Check sheet for the modelled part. Datum: model origin and axes. Units: mm. A direction names the side the tool comes from. Round coordinates to 2 decimals unless told otherwise and drop trailing zeros. Write each loop counter-clockwise with the first axis right and the second up, starting at its lowest first coordinate (ties: lowest second). Pieces come first, ordered by that corner, then holes.
Item 1: Section check A-A, the plane y = 0. Record the cut outline in (x, z).
Item 2: Set-up check for faces 4 (the flat face through (0, -23, 4)), 5 (the flat face through (4, 20, 4)), 6 (the flat face through (25.92, -14.11, -2.01)), 7 (the cylindrical face through (-25.148, 13.036, -1.93)): record each of +Z, -Z, +X, -X, +Y, -Y from which the full face is reachable in a straight line by a thin tool's end or side.
Item 3: Depth check by flat-ended pin: pin 1 (1.4 mm diameter, centred on y = -23, z = 2, fed in from -X); pin 2 (3.5 mm diameter, centred on x = -5.5, y = 21.5, fed in from -Z); pin 3 (5 mm diameter, centred on x = -3.5, y = -9.5, fed in from -Z); pin 4 (1.4 mm diameter, centred on x = 27.71, z = 1.7, fed in from -Y) (3 decimals). Enter the tip coordinate at first touch or a pass-through.
Item 4: Section check C-C, the plane z = -1.7. State how many separate pieces and enclosed holes the cut face has, plus the area to 3 significant figures.
Item 5: Release check for a two-part mould opening along Z. For faces 1 (the flat face through (5, 20, 6)), 2 (the cylindrical face through (-24.86, -13.036, 2.106)), 3 (the cylindrical face through (7.1, -17.6, 5)) record: pulls with the +Z half, pulls with the -Z half, needs draft (parallel to the pull), parting line crosses it, or undercut.
Item 6: Material ranges on line 1 along X through (y, z) = (13.5, -2); line 2 along X through (y, z) = (6, 0.25); line 3 along Y through (x, z) = (7.27, 5.6) (3 decimals), recorded low to high.
Item 7: Section check B-B, the plane x = -6.5. Record the cut outline in (y, z), plus the area to 3 significant figures.
from build123d import *

# Parameters (mm, degrees)
PAD_DEPTH       = 6.5
POCKET_DEPTH    = 6
SKETCH002_R     = 13.5
POCKET001_DEPTH = 1
SKETCH003_W     = 5.4
SKETCH003_H     = 6.5
PAD001_DEPTH    = 4.5
POCKET002_DEPTH = 10
SKETCH008_R     = 0.6
POCKET003_DEPTH = 2
SKETCH009_R     = 0.6
POCKET004_DEPTH = 2
FILLET_R        = 2.9
FILLET001_R     = 2.9
FILLET002_R     = 5
FILLET003_R     = 5
FILLET004_R     = 5
FILLET005_R     = 5
SKETCH010_W     = 3.95
SKETCH010_H     = 6.5
PAD002_DEPTH    = 4.5
POCKET005_DEPTH = 10
SKETCH012_R     = 0.6
POCKET006_DEPTH = 2
SKETCH013_R     = 0.6
POCKET007_DEPTH = 2
FILLET006_R     = 3.4
FILLET007_R     = 3.4
SKETCH014_R     = 20.45
SKETCH014_R_2   = 19.5
POCKET008_DEPTH = 0.3
SKETCH015_R     = 2.2
SKETCH015_R_2   = 0.975
PAD003_DEPTH    = 2
POCKET009_DEPTH = 4
POCKET010_DEPTH = 4
PAD004_DEPTH    = 3
CHAMFER_SIZE    = 2
CHAMFER001_SIZE = 2
CHAMFER002_SIZE = 2
CHAMFER003_SIZE = 2
SKETCH019_R     = 0.6
POCKET011_DEPTH = 2
SKETCH020_R     = 0.6
POCKET012_DEPTH = 2


with BuildPart() as part:
    # Sketch → Pad (new body)
    with BuildSketch(Plane.XY):
        with BuildLine():
            Line((-22.5019915649, 16), (-22.5019915649, -16))
            Line((-22.5019915649, -16), (-16.2858834577, -17.9000000001))
            ThreePointArc((-16.2858834577, -17.9000000001), (0.2206895737, -24.1989937004), (16.6096357576, -17.5999999999))
            Line((16.6096357576, -17.5999999999), (24.9082802252, -17.45))
            Line((24.9082802252, 17.45), (24.9082802252, -17.45))
            Line((16.6096357576, 17.6), (24.9082802252, 17.45))
            ThreePointArc((16.6096357576, 17.6), (0.2206895736, 24.1989937004), (-16.2858834578, 17.9))
            Line((-22.5019915649, 16), (-16.2858834578, 17.9))
        make_face()
    extrude(amount=PAD_DEPTH)

    # Sketch001 → Pocket (cut)
    with BuildSketch(Plane.XY):
        with BuildLine():
            Line((-14.8539557021, 16.9), (-21.2122180433, 15.55))
            Line((-21.2122180433, 15.55), (-21.2122180433, -15.55))
            Line((-21.2122180433, -15.55), (-14.8539557021, -16.9))
            ThreePointArc((-14.8539557021, -16.9), (-0.0760301383, -22.4998715423), (14.739402973, -17))
            Line((14.739402973, -17), (23.6191552218, -16.4))
            Line((23.6191552218, 16.4), (23.6191552218, -16.4))
            Line((14.739402973, 17), (23.6191552218, 16.4))
            ThreePointArc((14.739402973, 17), (-0.0760301383, 22.4998715423), (-14.8539557021, 16.9))
        make_face()
    extrude(amount=POCKET_DEPTH, mode=Mode.SUBTRACT)

    # Sketch002 (on Face19 of Pocket) → Pocket001 (cut)
    with BuildSketch(Plane(origin=(0, 0, 6), x_dir=(1, 0, 0), z_dir=(0, 0, -1))):
        Circle(SKETCH002_R)
    extrude(amount=-POCKET001_DEPTH, mode=Mode.SUBTRACT)

    # Sketch003 (on Face7 of Pad) → Pad001 (join)
    with BuildSketch(Plane.YZ.offset(24.9082802252)):
        with Locations((-14.75, 3.25)):
            Rectangle(SKETCH003_W, SKETCH003_H)
        with Locations((14.75, 3.25)):
            Rectangle(SKETCH003_W, SKETCH003_H)
    extrude(amount=PAD001_DEPTH)

    # Sketch006 (on Face22 of Pad001) → Pocket002 (cut)
    with BuildSketch(Plane.XY.offset(6.5)):
        with BuildLine():
            ThreePointArc((24.9082802252, 17.45), (26.9423471239, 15.7065020586), (29.4082802252, 14.6594169811))
            Line((29.4082802252, 17.45), (29.4082802252, 14.6594169811))
            Line((29.4082802252, 17.45), (24.9082802252, 17.45))
        make_face()
        with BuildLine():
            ThreePointArc((29.4082802252, -14.6594169811), (26.9423471239, -15.7065020586), (24.9082802252, -17.45))
            Line((29.4082802252, -17.45), (24.9082802252, -17.45))
            Line((29.4082802252, -14.6594169811), (29.4082802252, -17.45))
        make_face()
    extrude(amount=-POCKET002_DEPTH, mode=Mode.SUBTRACT)

    # Sketch008 (on Face27 of Pocket002) → Pocket003 (cut)
    with BuildSketch(Plane(origin=(0, -12.05, 0), x_dir=(-1, 0, 0), z_dir=(0, 1, 0))):
        with Locations((-27.7082802252, 1.7)):
            Circle(SKETCH008_R)
    extrude(amount=-POCKET003_DEPTH, mode=Mode.SUBTRACT)

    # Sketch009 (on Face26 of Pocket003) → Pocket004 (cut)
    with BuildSketch(Plane.XZ.offset(-12.05)):
        with Locations((27.7082802252, 1.7)):
            Circle(SKETCH009_R)
    extrude(amount=-POCKET004_DEPTH, mode=Mode.SUBTRACT)

    # Fillet
    fillet_edges = [part.edges().sort_by_distance(p)[0] for p in [
        (29.40828, -13.354708, 6.5),
    ]]
    fillet(fillet_edges, radius=FILLET_R)

    # Fillet001
    fillet001_edges = [part.edges().sort_by_distance(p)[0] for p in [
        (29.40828, 13.354708, 6.5),
    ]]
    fillet(fillet001_edges, radius=FILLET001_R)

    # Fillet002
    fillet002_edges = [part.edges().sort_by_distance(p)[0] for p in [
        (16.609636, -17.6, 3.25),
    ]]
    fillet(fillet002_edges, radius=FILLET002_R)

    # Fillet003
    fillet003_edges = [part.edges().sort_by_distance(p)[0] for p in [
        (16.609636, 17.6, 3.25),
    ]]
    fillet(fillet003_edges, radius=FILLET003_R)

    # Fillet004
    fillet004_edges = [part.edges().sort_by_distance(p)[0] for p in [
        (-16.285883, -17.9, 3.25),
    ]]
    fillet(fillet004_edges, radius=FILLET004_R)

    # Fillet005
    fillet005_edges = [part.edges().sort_by_distance(p)[0] for p in [
        (-16.285883, 17.9, 3.25),
    ]]
    fillet(fillet005_edges, radius=FILLET005_R)

    # Sketch010 (on Face3 of Pad) → Pad002 (join)
    with BuildSketch(Plane(origin=(-22.5019915649, 0, 0), x_dir=(0, -1, 0), z_dir=(-1, 0, 0))):
        with Locations((-14.025, 3.25)):
            Rectangle(SKETCH010_W, SKETCH010_H)
        with Locations((14.025, 3.25)):
            Rectangle(SKETCH010_W, SKETCH010_H)
    extrude(amount=PAD002_DEPTH)

    # Sketch011 (on Face6 of Pad002) → Pocket005 (cut)
    with BuildSketch(Plane.XY.offset(6.5)):
        with BuildLine():
            ThreePointArc((-27.0019915649, 14.6), (-24.6759937451, 15.0557212933), (-22.5019915649, 16))
            Line((-22.5019915649, 16), (-27.0019915649, 16))
            Line((-27.0019915649, 16), (-27.0019915649, 14.6))
        make_face()
        with BuildLine():
            ThreePointArc((-22.5019915649, -16), (-24.6759937451, -15.0557212933), (-27.0019915649, -14.6))
            Line((-27.0019915649, -14.6), (-27.0019915649, -16))
            Line((-27.0019915649, -16), (-22.5019915649, -16))
        make_face()
    extrude(amount=-POCKET005_DEPTH, mode=Mode.SUBTRACT)

    # Sketch012 (on Face23 of Pocket005) → Pocket006 (cut)
    with BuildSketch(Plane(origin=(0, -12.05, 0), x_dir=(-1, 0, 0), z_dir=(0, 1, 0))):
        with Locations((25.3019915649, 1.7)):
            Circle(SKETCH012_R)
    extrude(amount=-POCKET006_DEPTH, mode=Mode.SUBTRACT)

    # Sketch013 (on Face21 of Pocket006) → Pocket007 (cut)
    with BuildSketch(Plane.XZ.offset(-12.05)):
        with Locations((-25.3019915649, 1.7)):
            Circle(SKETCH013_R)
    extrude(amount=-POCKET007_DEPTH, mode=Mode.SUBTRACT)

    # Fillet006
    fillet006_edges = [part.edges().sort_by_distance(p)[0] for p in [
        (-27.001992, 13.325, 6.5),
    ]]
    fillet(fillet006_edges, radius=FILLET006_R)

    # Fillet007
    fillet007_edges = [part.edges().sort_by_distance(p)[0] for p in [
        (-27.001992, -13.325, 6.5),
    ]]
    fillet(fillet007_edges, radius=FILLET007_R)

    # Sketch014 (on Face4 of Fillet007) → Pocket008 (cut)
    with BuildSketch(Plane.XY.offset(6.5)):
        Circle(SKETCH014_R)
        Circle(SKETCH014_R_2, mode=Mode.SUBTRACT)
    extrude(amount=-POCKET008_DEPTH, mode=Mode.SUBTRACT)

    # Sketch015 (on Face55 of Pocket008) → Pad003 (join)
    with BuildSketch(Plane(origin=(0, 0, 6), x_dir=(1, 0, 0), z_dir=(0, 0, -1))):
        with Locations((-18.42, 13.32)):
            Circle(SKETCH015_R)
        with Locations((-18.42, 13.32)):
            Circle(SKETCH015_R_2, mode=Mode.SUBTRACT)
        with Locations((7.27, 18.56)):
            Circle(SKETCH015_R)
        with Locations((7.27, 18.56)):
            Circle(SKETCH015_R_2, mode=Mode.SUBTRACT)
        with Locations((5.37, -19.79)):
            Circle(SKETCH015_R)
        with Locations((5.37, -19.79)):
            Circle(SKETCH015_R_2, mode=Mode.SUBTRACT)
        with Locations((-18.42, -13.32)):
            Circle(SKETCH015_R)
        with Locations((-18.42, -13.32)):
            Circle(SKETCH015_R_2, mode=Mode.SUBTRACT)
    extrude(amount=PAD003_DEPTH)

    # Sketch016 → Pocket009 (cut)
    with BuildSketch(Plane(origin=(0, 0, 0), x_dir=(-1, 0, 0), z_dir=(0, 0, 1))):
        with BuildLine():
            Line((-5, 23.6778377391), (-5, 21.9374109685))
            ThreePointArc((5, 21.9374109685), (0, 22.5), (-5, 21.9374109685))
            Line((5, 23.6778377391), (5, 21.9374109685))
            ThreePointArc((5, 23.6778377391), (0, 24.2), (-5, 23.6778377391))
        make_face()
    extrude(amount=POCKET009_DEPTH, mode=Mode.SUBTRACT)

    # Sketch017 → Pocket010 (cut)
    with BuildSketch(Plane(origin=(0, 0, 0), x_dir=(-1, 0, 0), z_dir=(0, 0, 1))):
        with BuildLine():
            Line((-3.499984119, -22.2261132717), (-3.5, -23.9455632634))
            ThreePointArc((-3.5, -23.9455632634), (0, -24.2000019575), (3.5, -23.9455632634))
            Line((3.5000158811, -22.2261082701), (3.5, -23.9455632634))
            ThreePointArc((-3.499984119, -22.2261132717), (1.60767e-05, -22.5), (3.5000158811, -22.2261082701))
        make_face()
        with BuildLine():
            ThreePointArc((-13.9498796389, -17.6536358312), (-11.25, -19.4855715851), (-8.3135572795, -20.9077680626))
            Line((-8.3135572795, -20.9077680626), (-8.9416927184, -22.487466094))
            ThreePointArc((-15.0038705449, -18.987466094), (-12.1, -20.9578147716), (-8.9416927184, -22.487466094))
            Line((-13.9498796389, -17.6536358312), (-15.0038705449, -18.987466094))
        make_face()
        with BuildLine():
            ThreePointArc((8.3135572795, -20.9077680626), (11.25, -19.4855715851), (13.9498796389, -17.6536358312))
            Line((13.9498796389, -17.6536358312), (15.0038705449, -18.987466094))
            ThreePointArc((8.9416927184, -22.487466094), (12.1, -20.9578147716), (15.0038705449, -18.987466094))
            Line((8.3135572795, -20.9077680626), (8.9416927184, -22.487466094))
        make_face()
    extrude(amount=POCKET010_DEPTH, mode=Mode.SUBTRACT)

    # Sketch018 (on Face57 of Pocket010) → Pad004 (join)
    with BuildSketch(Plane(origin=(0, 0, 0), x_dir=(1, 0, 0), z_dir=(0, 0, -1))):
        with BuildLine():
            Line((29.4082802252, 14.6594169811), (29.4082802252, 12.05))
            Line((29.4082802252, 12.05), (24.9082802252, 12.05))
            Line((24.9082802252, 12.05), (24.9082802252, 17.45))
            ThreePointArc((24.9082802252, 17.45), (26.9423471239, 15.7065020586), (29.4082802252, 14.6594169811))
        make_face()
        with BuildLine():
            Line((29.4082802252, -12.05), (24.9082802252, -12.05))
            Line((24.9082802252, -17.45), (24.9082802252, -12.05))
            ThreePointArc((29.4082802252, -14.6594169811), (26.9423471239, -15.7065020586), (24.9082802252, -17.45))
            Line((29.4082802252, -12.05), (29.4082802252, -14.6594169811))
        make_face()
        with BuildLine():
            Line((-27.0019915649, 14.6), (-27.0019915649, 12.05))
            Line((-27.0019915649, 12.05), (-22.5019915649, 12.05))
            Line((-22.5019915649, 16), (-22.5019915649, 12.05))
            ThreePointArc((-27.0019915649, 14.6), (-24.6759937451, 15.0557212933), (-22.5019915649, 16))
        make_face()
        with BuildLine():
            Line((-27.0019915649, -12.05), (-22.5019915649, -12.05))
            Line((-22.5019915649, -12.05), (-22.5019915649, -16))
            ThreePointArc((-22.5019915649, -16), (-24.6759937451, -15.0557212933), (-27.0019915649, -14.6))
            Line((-27.0019915649, -12.05), (-27.0019915649, -14.6))
        make_face()
    extrude(amount=PAD004_DEPTH)

    # Chamfer
    chamfer_edges = [part.edges().sort_by_distance(p)[0] for p in [
        (-22.501992, -14.025, -3),
    ]]
    chamfer(chamfer_edges, length=CHAMFER_SIZE)

    # Chamfer001
    chamfer001_edges = [part.edges().sort_by_distance(p)[0] for p in [
        (-22.501992, 14.025, -3),
    ]]
    chamfer(chamfer001_edges, length=CHAMFER001_SIZE)

    # Chamfer002
    chamfer002_edges = [part.edges().sort_by_distance(p)[0] for p in [
        (24.90828, -14.75, -3),
    ]]
    chamfer(chamfer002_edges, length=CHAMFER002_SIZE)

    # Chamfer003
    chamfer003_edges = [part.edges().sort_by_distance(p)[0] for p in [
        (24.90828, 14.75, -3),
    ]]
    chamfer(chamfer003_edges, length=CHAMFER003_SIZE)

    # Sketch019 (on Face5 of Chamfer003) → Pocket011 (cut)
    with BuildSketch(Plane.XZ.offset(-12.05)):
        with Locations((28.1082802252, -1.7)):
            Circle(SKETCH019_R)
        with Locations((-25.7019915649, -1.7)):
            Circle(SKETCH019_R)
    extrude(amount=-POCKET011_DEPTH, mode=Mode.SUBTRACT)

    # Sketch020 (on Face83 of Pocket011) → Pocket012 (cut)
    with BuildSketch(Plane(origin=(0, -12.05, 0), x_dir=(-1, 0, 0), z_dir=(0, 1, 0))):
        with Locations((25.7019915649, -1.7)):
            Circle(SKETCH020_R)
        with Locations((-28.1082802252, -1.7)):
            Circle(SKETCH020_R)
    extrude(amount=-POCKET012_DEPTH, mode=Mode.SUBTRACT)


solid = part.part
Values found:
1. outline: (-22.5, 0) - (-21.21, 0) - (-21.21, 6) - (-13.5, 6) - (-13.5, 6.5) - (-19.5, 6.5) - (-19.5, 6.2) - (-20.45, 6.2) - (-20.45, 6.5) - (-22.5, 6.5) - close; (13.5, 6) - (23.62, 6) - (23.62, 0) - (24.91, 0) - (24.91, 6.5) - (20.45, 6.5) - (20.45, 6.2) - (19.5, 6.2) - (19.5, 6.5) - (13.5, 6.5) - close
2. face 4: -Z, -Y
2. face 5: -Z
2. face 6: -Z, +Y, -Y
2. face 7: none
3. pin 1: stops at x = -9.4
3. pin 2: stops at z = 0
3. pin 3: passes through
3. pin 4: stops at y = -15.665
4. separate pieces: 4
4. enclosed holes: 0
4. area: 38.9 mm2
5. face 1: pulls with the -Z half
5. face 2: undercut
5. face 3: needs draft
6. line 1: x = -27 to -26.22, -25.18 to -23.5, 25.91 to 27.59, 28.63 to 29.41
6. line 2: x = -22.5 to -21.21, 23.62 to 24.91
6. line 3: y = -23.082 to -21.293, -20.76 to -19.535, -17.585 to -16.36, 18.681 to 20.899, 21.293 to 23.082
7. outline: (-23.31, 0) - (-21.54, 0) - (-21.54, 6) - (-11.83, 6) - (-11.83, 6.5) - (-18.38, 6.5) - (-18.38, 6.2) - (-19.39, 6.2) - (-19.39, 6.5) - (-23.31, 6.5) - close; (11.83, 6) - (21.54, 6) - (21.54, 0) - (23.31, 0) - (23.31, 6.5) - (19.39, 6.5) - (19.39, 6.2) - (18.38, 6.2) - (18.38, 6.5) - (11.83, 6.5) - close
7. area: 32.1 mm2
